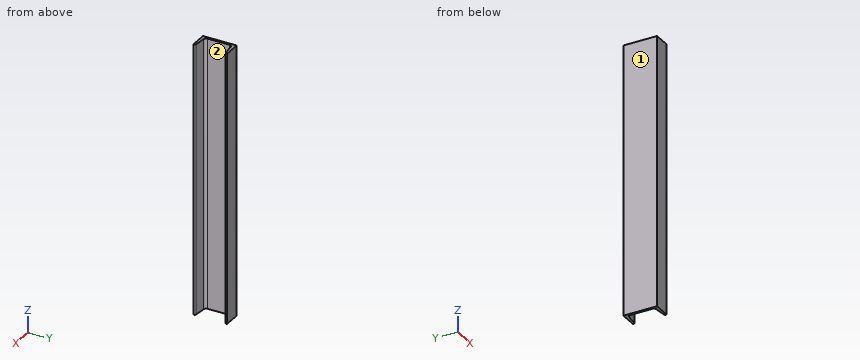
Autodesk Inventor part; units mm, degrees
ref_plane "Start Plane" through (0, 0, 0) normal (0, 0, 1) x (1, 0, 0)
ref_plane "End Plane" through (0, 0, 800) normal (0, 0, 1) x (1, 0, 0)
ref_plane "YZ Plane" through (0, 0, 0) normal (1, 0, 0) x (0, 1, 0)
ref_plane "Start Plane" through (0, 0, 0) normal (0, 0, 1) x (1, 0, 0)
ref_plane "End Plane" through (0, 0, 800) normal (0, 0, 1) x (1, 0, 0)
sketch "Sketch" plane through (0, 0, 0) normal (0, 0, 1) x (1, 0, 0)
  line L0 (-1.51, 0) -> (-1.51, 50)
  line L1 (-1.51, 50) -> (48.49, 50)
  line L2 (48.49, 50) -> (48.49, 48.3694)
  line L3 (44.4604, 43.894) -> (11.5538, 40.4354)
  line L4 (4.39, 32.4792) -> (4.39, 0)
  line L5 (4.39, 0) -> (-1.51, 0) construction
  line L6 (26.44, 50) -> (26.44, 42) construction
  line L7 (48.49, 44.3175) -> (48.49, 42) construction
  line L8 (48.49, 42) -> (26.44, 42) construction
  line L9 (0, 15) -> (0, -27) construction
  line L10 (-5.539, 0) -> (16.0067, 0) construction
  line L11 (-1.51, 0) -> (-1.51, -50)
  line L12 (-1.51, -50) -> (48.49, -50)
  line L13 (48.49, -50) -> (48.49, -48.3694)
  line L14 (44.4604, -43.894) -> (11.5538, -40.4354)
  line L15 (4.39, -32.4792) -> (4.39, 0)
  arc A0 (11.5538, 40.4354) -> (4.39, 32.4792) centre (12.39, 32.4792) ccw
  arc A1 (4.39, -32.4792) -> (11.5538, -40.4354) centre (12.39, -32.4792) ccw
  arc A2 (44.4604, 43.894) -> (48.49, 48.3694) centre (43.99, 48.3694) ccw
  arc A3 (48.49, -48.3694) -> (44.4604, -43.894) centre (43.99, -48.3694) ccw
  line L16 (0, 70) -> (0, -70) construction
  line L17 (-16.5166, 0) -> (60.3266, 0) construction
  point P0 (4.39, 39.6825)
  point P1 (48.49, -44.3175)
  point P2 (4.39, -39.6825)
  point P3 (26.44, -50)
  point P4 (26.44, -42)
  dimension "d0" = 5.9
  dimension "d1" = 50
  dimension "d2" = 50
  dimension "d3" = 8
  dimension "d4" = 22.05
  dimension "d5" = 2.3175
  dimension "d23" = 8
  dimension "d24" = 4.5
  dimension "d25" = 1.51
extrude "Body" add sketch "Sketch" along normal up to surface (800 mm away) from surface at 0
sketch "Sketch3" plane through (0, 0, 0) normal (0, 0, 1) x (1, 0, 0)
  line L0 (0, 0) -> (10, 0)
ref_plane "Work Plane3" through (0, 0, 0) normal (0, -1, 0) x (1, 0, 0)
sketch "Sketch4" plane through (0, 0, 0) normal (0, -1, 0) x (1, 0, 0)
  line L0 (-2, 0) -> (12, 0)
  line L1 (-2, 800) -> (12, 800)
  dimension "d29" = 800
equation "\"d0\" = G_T"
equation "\"d1\" = 0.5 * G_H"
equation "\"d2\" = G_W"
equation "\"d3\" = G_T1"
equation "\"d4\" = G_C"
equation "\"d23\" = G_IR"
equation "\"d24\" = G_ER"
equation "\"d25\" = ex"
equation "\"d6\" = G_L"
equation "\"G_W\" = 50"
equation "\"G_H\" = 100"
equation "\"G_T\" = 5.9"
equation "\"G_T1\" = 8"
equation "\"G_NG\" = 0.105104"
equation "\"G_ER\" = 4.5"
equation "\"G_IR\" = 8"
equation "\"G_C\" = 22.05"
equation "\"G_L\" = d29"
equation "\"ex\" = 1.51"
equation "\"G_OFFSET_START\" = 0"
equation "\"G_OFFSET_END\" = 0"
properties part number "ISO 657_11 CH 100 x 10 1744276061340" material "Steel, Mild"
The listing builds one solid part. Answer for the finished solid, in the listing's coordinates (mm). Face numbers are marked on the shaded views. Coordinates: 2 decimals unless noted, no trailing zeros. Write each loop counter-clockwise with the first axis right and the second up, starting at its lowest first coordinate (ties: lowest second). Pieces come first, ordered by that corner, then holes. Notation, with made-up numbers: (1.5, 58.25) - (14.5, 58.25) arc R17 cw to (14.5, 79.25) - close; hole circle Ø7 at (19, 15.25). An arc over 180 degrees is marked (long way). Return JSON: item names as keys, results as strings. Group by question number.
Q1. The part is cut by section A-A on x = 20. Write down the section's boundary in (y, z), and give its area (3 significant figures).
Q2. Flat-ended cylindrical pins translate along their axes: pin 1 Ø6 at (x, y) = (10, -13) entering from -Z; pin 2 Ø2 at (y, z) = (22.5, 166.5) entering from +X. Find the tip coordinate at first contact, or state that the pin passes through.
Q3. The part is cut by section C-C on y = -19. Write down the section's boundary in (x, z).
Q4. Find the intervals of material crossed by line 1 along X through (y, z) = (2.5, 162); line 2 along Y through (x, z) = (9.5, 741); line 3 along Y through (x, z) = (5, 359), in increasing order. Write a range as [from, to].
Q5. For a pull along Y with two mould halves and no side action, classify the marked faces 1 and 2 as +Y half, -Y half, draft (parallel to the pull), parting line (faces both ways), or undercut.
Q6. The part is cut by section B-B on z = 523. Write down the section's boundary in (x, y).
Evaluation:
{
 "1": {"outline": "(-50, 0) - (-41.32, 0) - (-41.32, 800) - (-50, 800) - close; (41.32, 0) - (50, 0) - (50, 800) - (41.32, 800) - close", "area": "13,900 mm2"},
 "2": {"pin 1": "passes through", "pin 2": "stops at x = 4.39"},
 "3": {"outline": "(-1.51, 0) - (4.39, 0) - (4.39, 800) - (-1.51, 800) - close"},
 "4": {"line 1": "x = [-1.51, 4.39]", "line 2": "y = [-50, -39.94], [39.94, 50]", "line 3": "y = [-50, -35.54], [35.54, 50]"},
 "5": {"face 1": "draft", "face 2": "undercut"},
 "6": {"outline": "(-1.51, -50) - (48.49, -50) - (48.49, -48.37) arc R4.5 ccw to (44.46, -43.89) - (11.55, -40.44) arc R8 cw to (4.39, -32.48) - (4.39, 32.48) arc R8 cw to (11.55, 40.44) - (44.46, 43.89) arc R4.5 ccw to (48.49, 48.37) - (48.49, 50) - (-1.51, 50) - close"}
}
